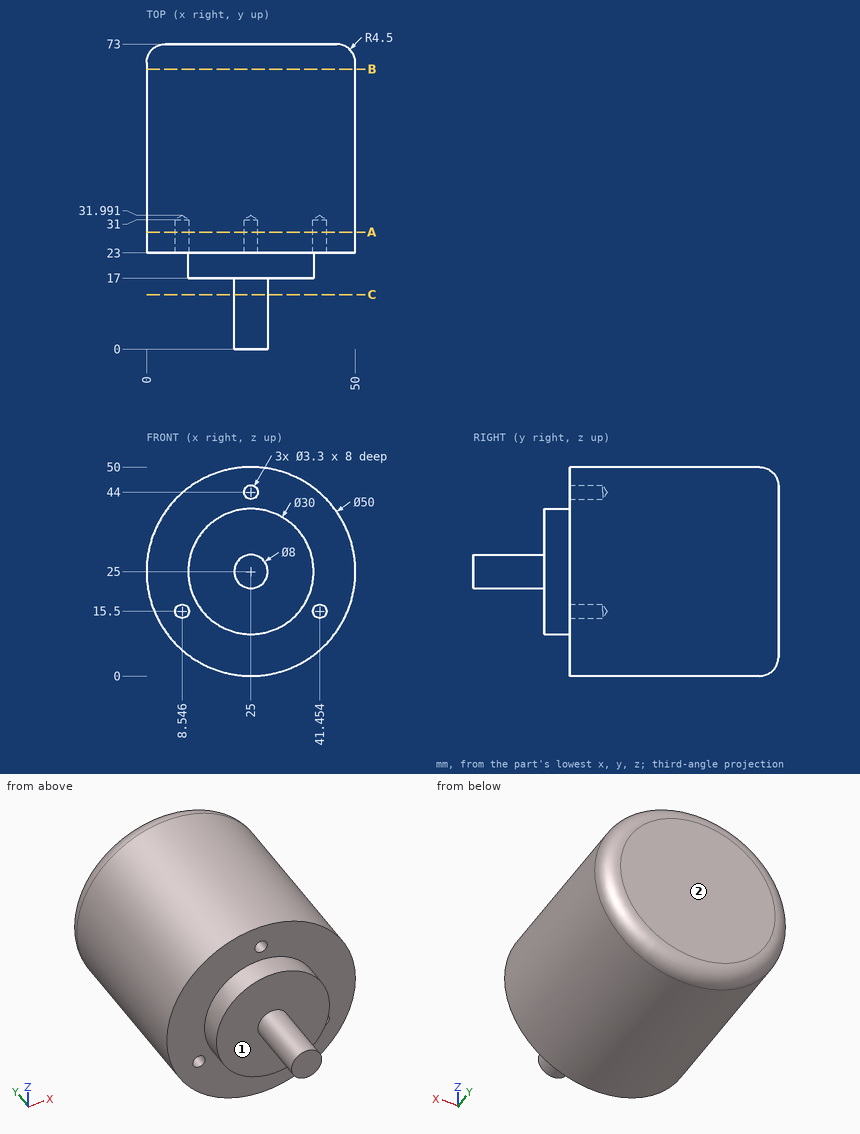
Input: dimensioned drawing with shaded views. Units: mm. Origin: part minimum x, y, z. A direction names the side the tool comes from. Give positions to 0.01 mm unless a question says otherwise; leave off trailing zeros. Write each loop counter-clockwise with the first axis right and the second up, starting at its lowest first coordinate (ties: lowest second). Pieces come first, ordered by that corner, then holes.
Q1. Section A-A, the plane y = 28. State how many separate pieces and enclosed holes the cut face has, plus the area to 3 significant figures.
Q2. Section C-C, the plane y = 13. Output: boundary loops of the cut face in (x, z).
Q3. Section B-B, the plane y = 67. Output: boundary loops of the cut face in (x, z), plus the area to 3 significant figures.
Q4. Set-up query: the marked faces 1 and 2. Return all of +Z, -Z, +X, -X, +Y, -Y with unobstructed straight access to the full face (end or side cutting, diameter ignored); none if empty.
Q5. First-contact query: P1, Ø24, axis at x = 23.5, z = 20.5, coming from the -Y side; P2, Ø3, axis at x = 25, z = 44, coming from the -Y side; P3, Ø6, axis at y = 58, z = 28.5, coming from the +X side (1 decimal); P4, Ø4, axis at x = 8.55, z = 15.5, coming from the -Y side. Flat tips, straight axial feed; report the tip coordinate or a pass-through.
Q6. Material intervals for probe 1 along X at (y, z) = (28, 15); probe 2 along Z at (x, y) = (25, 29); probe 3 along Y at (x, z) = (8, 13.5), sorted ascending.
Filled in:
1. separate pieces: 1
1. enclosed holes: 3
1. area: 1,940 mm2
2. outline: circle Ø8 at (25, 25)
3. outline: circle Ø50 at (25, 25)
3. area: 1,960 mm2
4. face 1: -Y
4. face 2: +Z, -Z, +X, -X, +Y
5. P1: stops at y = 0
5. P2: stops at y = 31.09
5. P3: stops at x = 50
5. P4: stops at y = 23
6. probe 1: x = 2.09 to 6.97, 10.12 to 39.88, 43.03 to 47.91
6. probe 2: z = 0 to 42.35, 45.65 to 50
6. probe 3: y = 23 to 73
